For this review, use the dimensioned drawing (mm, ordinates from the lowest corner) and the shaded views. A direction names the side the tool comes from. Give positions to 0.01 mm unless a question says otherwise; leave off trailing zeros. Order: outer loops, then holes, each group sorted by start corner. A loop starts at its lowest first (then second) coordinate and runs counter-clockwise, first axis right, second up. Notation, with made-up numbers: (4, 59) - (58, 59) arc R16 cw to (58, 70) - close; hole circle Ø7 at (61.5, 59). An arc over 180 degrees is marked (long way). Use a Markdown table: item, result. Add a question column.
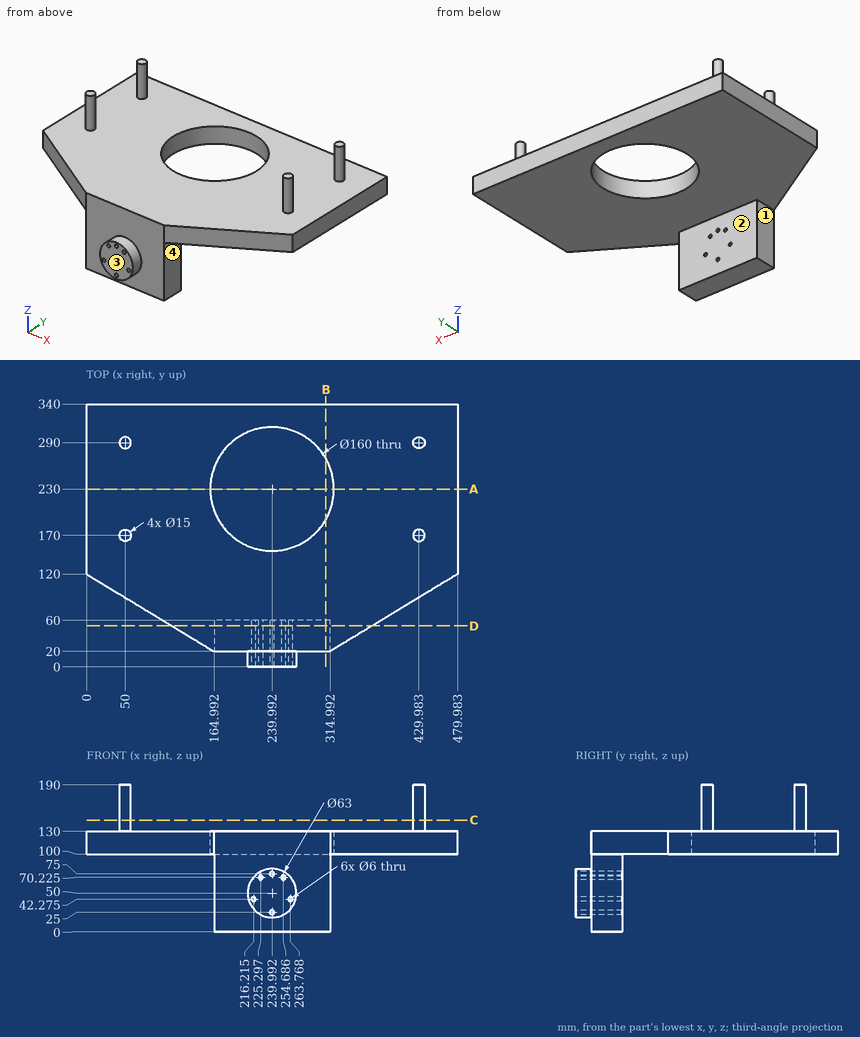
Q1. Machinability: for the marked faces 1, 2, 3 and 4, which of the approach directions +Z, -Z, +X, -X, +Y, -Y give a long, thin tool a straight path to every point of the face, cutting with its end or side? Answer none if there is none.
Q2. Clearance check with flat-ended pins moving along their axes: P1, Ø5.5, axis at x = 216.22, z = 42.27, coming from the -Y side; P2, Ø20, axis at y = 30, z = 69, coming from the -X side; P3, Ø8, axis at x = 296, y = 125.5, coming from the +Z side. State where each tip first meets the part, or that it passes through.
Q3. We need section C-C (z = 144.5). Write out the cut boundary in (x, y).
Q4. We need section A-A (y = 230). Write out the cut boundary in (x, z).
Q5. Wall thickness on probe 1 along X at (y, z) = (169.5, 143); probe 2 along Z at (x, y) = (364, 160.5); probe 3 along Y at (x, z) = (295, 87): over which ranges is each line inside the solid? List them lowest first.
Q6. We need section B-B (x = 309.5). Write out the cut boundary in (y, z) (1 decimal), plus the area to 3 significant figures.
Q7. We need section D-D (y = 53). Write out the cut boundary in (x, z) (1 decimal), plus the area to 3 significant figures.
Here are the results:
| question | item | result |
|---|---|---|
| 1 | face 1 | -Z, -X, +Y, -Y |
| 1 | face 2 | -Z, +X, -X, +Y |
| 1 | face 3 | +Z, -Z, +X, -X, -Y |
| 1 | face 4 | -Z, +X, +Y, -Y |
| 2 | P1 | through |
| 2 | P2 | x = 164.99 |
| 2 | P3 | z = 130 |
| 3 | outline | circle Ø15 at (50, 170); circle Ø15 at (50, 290); circle Ø15 at (429.98, 170); circle Ø15 at (429.98, 290) |
| 4 | outline | (0, 100) - (159.99, 100) - (159.99, 130) - (0, 130) - close; (319.99, 100) - (479.98, 100) - (479.98, 130) - (319.99, 130) - close |
| 5 | probe 1 | 42.52 to 57.48, 422.5 to 437.47 |
| 5 | probe 2 | 100 to 130 |
| 5 | probe 3 | 20 to 60 |
| 6 | outline | (20, 0) - (60, 0) - (60, 100) - (190.4, 100) - (190.4, 130) - (20, 130) - close; (269.6, 100) - (340, 100) - (340, 130) - (269.6, 130) - close |
| 6 | area | 11,200 mm2 |
| 7 | outline | (110.5, 100) - (165, 100) - (165, 0) - (315, 0) - (315, 100) - (369.4, 100) - (369.4, 130) - (110.5, 130) - close; hole circle Ø6 at (216.2, 42.3); hole circle Ø6 at (225.3, 70.2); hole circle Ø6 at (240, 25); hole circle Ø6 at (240, 75); hole circle Ø6 at (254.7, 70.2); hole circle Ø6 at (263.8, 42.3) |
| 7 | area | 22,600 mm2 |
